CAD build for the part. Positions are in the model's coordinates, mm. A direction names the side the tool comes from. Coordinates: 2 decimals unless noted, no trailing zeros. Loops run counter-clockwise (first coordinate to the right, second up) from the corner with the lowest first, then second, coordinate; pieces in that order, holes last. Notation, with made-up numbers: (-14, 70.25) -> (40, 70.25) arc R23 ccw to (40, 104.25) -> close; hole circle Ø6 at (-17.5, 53.5). An arc over 180 degrees is marked (long way). Answer as a JSON object with one key per item and string values. Group by question number.
from build123d import *

# Parameters (mm, degrees)
BOX001_W                  = 20
BOX001_H                  = 10
BOX001_DEPTH              = 20
BOX002_W                  = 10
BOX002_H                  = 20
BOX002_DEPTH              = 10
BOX003_W                  = 10
BOX003_H                  = 10
BOX003_DEPTH              = 10
BOX004_W                  = 30
BOX004_H                  = 10
BOX004_DEPTH              = 10
BOX005_W                  = 10
BOX005_H                  = 20
BOX005_DEPTH              = 20
BOX006_W                  = 10
BOX006_H                  = 30
BOX006_DEPTH              = 10
BOX007_W                  = 10
BOX007_H                  = 10
BOX007_DEPTH              = 10
BOX_W                     = 10
BOX_H                     = 10
BOX_DEPTH                 = 30
FUSION001_PLACEMENT_ANGLE = 337.5


with BuildPart() as cub001:
    # Box001 → Box001 (new body)
    with BuildSketch(Plane.XY):
        with Locations((10, 5)):
            Rectangle(BOX001_W, BOX001_H)
    extrude(amount=BOX001_DEPTH)


with BuildPart() as cub002:
    # Box002 → Box002 (new body)
    with BuildSketch(Plane.XY):
        with Locations((5, 10)):
            Rectangle(BOX002_W, BOX002_H)
    extrude(amount=BOX002_DEPTH)


with BuildPart() as cub003:
    # Box003 → Box003 (new body)
    with BuildSketch(Plane.XY):
        with Locations((5, 5)):
            Rectangle(BOX003_W, BOX003_H)
    extrude(amount=BOX003_DEPTH)


with BuildPart() as cub004:
    # Box004 → Box004 (new body)
    with BuildSketch(Plane.XY):
        with Locations((15, 5)):
            Rectangle(BOX004_W, BOX004_H)
    extrude(amount=BOX004_DEPTH)


with BuildPart() as cub005:
    # Box005 → Box005 (new body)
    with BuildSketch(Plane.XY):
        with Locations((5, 10)):
            Rectangle(BOX005_W, BOX005_H)
    extrude(amount=BOX005_DEPTH)


with BuildPart() as cub006:
    # Box006 → Box006 (new body)
    with BuildSketch(Plane.XY):
        with Locations((5, 15)):
            Rectangle(BOX006_W, BOX006_H)
    extrude(amount=BOX006_DEPTH)


with BuildPart() as cub007:
    # Box007 → Box007 (new body)
    with BuildSketch(Plane(origin=(10, 10, 0), x_dir=(1, 0, 0), z_dir=(0, 0, 1))):
        with Locations((5, 5)):
            Rectangle(BOX007_W, BOX007_H)
    extrude(amount=BOX007_DEPTH)


with BuildPart() as fusion001:
    # Box → Box (new body)
    with BuildSketch(Plane.XY):
        with Locations((5, 5)):
            Rectangle(BOX_W, BOX_H)
    extrude(amount=BOX_DEPTH)

    # Fusion: union Cub001, Cub002, Cub003, Cub004, Cub005, Cub006, Cub007
    add(cub001.part)
    add(cub002.part)
    add(cub003.part)
    add(cub004.part)
    add(cub005.part)
    add(cub006.part)
    add(cub007.part)


with BuildPart() as fusion001_1:
    # Fusion001 placement: moved
    add(fusion001.part.moved(Location((-13.858193, -5.740251, 0))).rotate(Axis((-13.858193, -5.740251, 0), (0, 0, 1)), FUSION001_PLACEMENT_ANGLE))


solid = fusion001_1.part
Item 1: Drill centre lines: L1, parallel to Z at x = 6, y = 6; L2, parallel to Y at x = 5, z = 8.75; L3, parallel to Y at x = 3.5, z = 1.75. Where is each one in solid material? Low to high.
Item 2: Band-saw the part on A-A, the plane x = 10. List the corners of the cut face in (y, z), and give its area (3 significant figures).
Item 3: Band-saw the part on D-D, the plane y = 10. List the corners of the cut face in (x, z).
Item 4: Band-saw the part on B-B, the plane z = 8.5. List the corners of the cut face in (x, y), and give its area (3 significant figures).
Item 5: Flat gauge pins, fed straight in: P1, Ø4, axis at x = 1.5, y = 17.5, coming from the +Z side; P2, Ø14.5, axis at x = 13, y = -11.5, coming from the +Z side; P3, Ø10, axis at x = -9.5, z = 11.5, coming from the -Y side. Where does each tip first touch, or does it go through?
Item 6: Band-saw the part on C-C, the plane x = -9. List the corners of the cut face in (y, z).
Item 7: 3-axis set-ups, long thin cutter, end or side, ignore diameter. For faces 1 (the flat face through (13, -6.04, 4.93)), 2 (the flat face through (6, 2, 10)), 3 (the flat face through (-5.477, 1.612, 24.93)), 4 (the flat face through (2, -7, 20)): which of +Z, -Z, +X, -X, +Y, -Y reach the whole face in a straight line?
Reply:
{
 "1": {"L1": "0 to 10", "L2": "-13.55 to 8.1, 13.66 to 18.92", "L3": "-12.93 to 8.72, 10.03 to 19.54"},
 "2": {"outline": "(-15.62, 0) -> (-4.8, 0) -> (-4.8, 10) -> (-15.62, 10) -> close; (-0.4, 0) -> (6.03, 0) -> (6.03, 10) -> (-0.4, 10) -> close", "area": "173 mm²"},
 "3": {"outline": "(-7.34, 0) -> (3.49, 0) -> (3.49, 10) -> (0.4, 10) -> (0.4, 20) -> (-7.34, 20) -> close"},
 "4": {"outline": "(-13.86, -5.74) -> (13.86, -17.22) -> (17.69, -7.98) -> (8.45, -4.16) -> (12.27, 5.08) -> (3.03, 8.91) -> (6.86, 18.15) -> (-2.38, 21.98) -> close", "area": "600 mm²"},
 "5": {"P1": "z = 10", "P2": "z = 20", "P3": "y = -9.62"},
 "6": {"outline": "(-7.75, 0) -> (5.99, 0) -> (5.99, 20) -> (3.07, 20) -> (3.07, 30) -> (-7.75, 30) -> close"},
 "7": {"face 1": "+Z, -Z, +X", "face 2": "+Z, +X", "face 3": "+Z, +X, +Y", "face 4": "+Z, +X, -Y"}
}
